The listing builds one solid part. Answer for the finished solid, in the listing's coordinates (mm). A direction names the side the tool comes from. Coordinates: 2 decimals unless noted, no trailing zeros. Order: outer loops, then holes, each group sorted by start corner. A loop starts at its lowest first (then second) coordinate and runs counter-clockwise, first axis right, second up. Notation, with made-up numbers: (-19.5, -31) -> (37.5, -31) arc R28 cw to (37.5, -10) -> close; hole circle Ø10 at (48.25, 72). An arc over 180 degrees is marked (long way). Write each question's results on one line, items separated by ' | '. Start each with the question number.
(1) The part is cut by section B-B, the plane y = 0. Give the vertices of the cut face in (x, z).
(2) The part is cut by section C-C, the plane x = 0. Give the vertices of the cut face in (y, z).
(3) The part is cut by section D-D, the plane y = -25. Give the vertices of the cut face in (x, z).
(4) Straight lines are drawn through the part: L1, parallel to Z at x = -24.5, y = 20.5; L2, parallel to X at y = 15.5, z = -31.5; L3, parallel to Y at x = 46, z = 3.5. For each, find the intervals that lie inside material, in ascending order.
(5) The part is cut by section A-A, the plane z = 7. Give the vertices of the cut face in (x, y), then the cut area to 3 significant figures.
(6) Given pin 1 (8 mm diameter, centred on x = -19.5, z = 66.5, fed in from -Y) (3 decimals); pin 2 (5 mm diameter, centred on x = -14, z = 66.5, fed in from -Y); pin 3 (1.5 mm diameter, centred on y = 0.5, z = 49, fed in from -X), each flat-ended and moving along its own axis, determine where each tip first touches the part or whether it passes through.
(7) A tool of negligible diameter and unlimited length cuts with its end or side. For faces 1 (the face through (-37.81, 54.81, -32.44)), 2 (the face through (-16.11, -12.35, 65.7)), from which of +Z, -Z, +X, -X, +Y, -Y can it reach the whole face along a straight path? Write none if from no direction.
```python
from build123d import *

# Parameters (mm, degrees)
F0_W     = 101.289254
F0_H     = 69.795959
F1_DEPTH = 63.5
F2_SIZE  = 12.7
F3_R     = 20.297571
F4_DEPTH = 73.406


with BuildPart() as f1:
    # F0 (on Front) → F1 (new body, symmetric)
    with BuildSketch(Plane.XZ):
        with Locations((3.972126, -5.390744)):
            Rectangle(F0_W, F0_H)
    extrude(amount=F1_DEPTH, both=True)

    # F2
    f2_edges = [f1.edges().sort_by_distance(p)[0] for p in [
        (3.972126, -63.5, 29.507235),
        (54.616753, 0, 29.507235),
        (3.972126, 63.5, 29.507235),
        (-46.672501, 0, 29.507235),
        (54.616753, -63.5, -5.390745),
        (54.616753, 63.5, -5.390745),
        (-46.672501, -63.5, -5.390745),
        (-46.672501, 63.5, -5.390745),
        (3.972126, 63.5, -40.288724),
        (-46.672501, 0, -40.288724),
        (3.972126, -63.5, -40.288724),
        (54.616753, 0, -40.288724),
    ]]
    chamfer(f2_edges, length=F2_SIZE)

    # F3 (on face) → F4 (join)
    with BuildSketch(Plane.XY.offset(29.507235)):
        Circle(F3_R)
    extrude(amount=F4_DEPTH)


solid = f1.part
```
Established:
1) outline: (-46.67, -27.59) -> (-33.97, -40.29) -> (41.92, -40.29) -> (54.62, -27.59) -> (54.62, 16.81) -> (41.92, 29.51) -> (20.3, 29.51) -> (20.3, 102.91) -> (-20.3, 102.91) -> (-20.3, 29.51) -> (-33.97, 29.51) -> (-46.67, 16.81) -> close
2) outline: (-63.5, -27.59) -> (-50.8, -40.29) -> (50.8, -40.29) -> (63.5, -27.59) -> (63.5, 16.81) -> (50.8, 29.51) -> (20.3, 29.51) -> (20.3, 102.91) -> (-20.3, 102.91) -> (-20.3, 29.51) -> (-50.8, 29.51) -> (-63.5, 16.81) -> close
3) outline: (-46.67, -27.59) -> (-33.97, -40.29) -> (41.92, -40.29) -> (54.62, -27.59) -> (54.62, 16.81) -> (41.92, 29.51) -> (-33.97, 29.51) -> (-46.67, 16.81) -> close
4) L1: z = -40.29 to 29.51 | L2: x = -42.76 to 50.71 | L3: y = -59.42 to 59.42
5) outline: (-46.67, -50.8) -> (-33.97, -63.5) -> (41.92, -63.5) -> (54.62, -50.8) -> (54.62, 50.8) -> (41.92, 63.5) -> (-33.97, 63.5) -> (-46.67, 50.8) -> close | area: 12,500 mm^2
6) pin 1: stops at y = -13.105 | pin 2: stops at y = -16.73 | pin 3: stops at x = -20.3
7) face 1: -Z, -X, +Y | face 2: +Z
